Model file for the job. Use its own axes, mm. A direction names the side the tool comes from. Round coordinates to 2 decimals unless told otherwise and drop trailing zeros. Order: outer loops, then holes, each group sorted by start corner. A loop starts at its lowest first (then second) coordinate and runs counter-clockwise, first axis right, second up. Notation, with made-up numbers: (-12, 74) - (9, 74) arc R22 ccw to (9, 106) - close; hole circle Ø11 at (76, -14.75). An arc over 180 degrees is marked (long way). Put each result on its own line as item: value. Start each with the question number.
Item 1: Which spindle directions (+Z, -Z, +X, -X, +Y, -Y) get a long thin tool onto all of the face, cutting with end or side? Do faces 1 (the face through (-10, -43, -68)), 2 (the face through (-47, -27, -50)), 3 (the face through (-44.863, -37.283, 48.623)). Say none if no direction does.
Item 2: Pin check, flat tips, straight feed: pin 1 Ø5 at (x, z) = (-24, -45) entering from +Y; pin 2 Ø8 at (x, y) = (-36, -60) entering from +Z; pin 3 Ø1.5 at (x, y) = (-22.5, -65.5) entering from -Z. Stop position of each tip, or through.
Item 3: Probe probe 1 along Z at (x, y) = (-45, 2); probe 2 along X at (y, z) = (-60, -56); probe 3 along Y at (x, z) = (-3.5, -26). List the from-to ranges inside material, lowest first.
Item 4: Saw through at A-A on x = -17. List the corners of the cut face in (y, z), plus the area to 3 significant figures.
```python
from build123d import *


with BuildPart() as part:
    # OutRacSke → OuterRace (revolve)
    with BuildSketch(Plane.XY, mode=Mode.PRIVATE) as outerrace_sk:
        with BuildLine():
            Line((-10, 79.990044662), (-47, 73.1325))
            Line((-47, 73.1325), (-47, 83))
            ThreePointArc((-47, 83), (-46.414213562, 84.414213562), (-45, 85))
            Line((-45, 85), (-11.48, 85))
            Line((-11.48, 85), (-10, 83.52))
            Line((-10, 83.52), (-10, 79.990044662))
        make_face()
    revolve(outerrace_sk.sketch.rotate(Axis((-42.5, 0, 0), (1, 0, 0)), 270), axis=Axis((-42.5, 0, 0), (1, 0, 0)))

    # RolSimSke → RollersSimplified (revolve)
    with BuildSketch(Plane.XY, mode=Mode.PRIVATE) as rollerssimplified_sk:
        Polygon((-45, 73.87069398), (-12.257611578, 79.939136979), (-9.797431984, 66.665195727), (-42.539820406, 60.596752728), align=None)
    revolve(rollerssimplified_sk.sketch.rotate(Axis((0, 0, 0), (-1, 0, 0)), 90), axis=Axis((0, 0, 0), (-1, 0, 0)))

    # InsRacSke → InnerRace (revolve)
    with BuildSketch(Plane.XY, mode=Mode.PRIVATE) as innerrace_sk:
        with BuildLine():
            Line((-42.652623366, 61.271752727), (-47, 61.271752727))
            Line((-47, 61.271752727), (-47, 56.48))
            Line((-47, 56.48), (-45.52, 55))
            Line((-45.52, 55), (-2.5, 55))
            ThreePointArc((-2.5, 55), (-0.732233047, 55.732233047), (0, 57.5))
            Line((0, 57.5), (0, 68.015195726))
            Line((0, 68.015195726), (-9.785131089, 68.015195726))
            Line((-9.785131089, 68.015195726), (-9.785131089, 66.665195726))
            Line((-9.785131089, 66.665195726), (-42.527519511, 60.596752727))
            Line((-42.527519511, 60.596752727), (-42.652623366, 61.271752727))
        make_face()
    revolve(innerrace_sk.sketch.rotate(Axis((-42.5, 0, 0), (1, 0, 0)), 270), axis=Axis((-42.5, 0, 0), (1, 0, 0)))


solid = part.part
```
Results found:
1. face 1: +X
1. face 2: +Z, -Z, -X, +Y, -Y
1. face 3: -X
2. pin 1: stops at y = 73.61
2. pin 2: stops at z = 63.95
2. pin 3: stops at z = -55.07
3. probe 1: z = -84.98 to -73.48, -61.24 to -54.96, 54.96 to 61.24, 73.48 to 84.98
3. probe 2: x = -47 to -10
3. probe 3: y = -62.85 to -48.47, 48.47 to 62.85
4. outline: circle Ø170 at (0, 0); circle Ø130.66 at (0, 0); hole circle Ø130.66 at (0, 0); hole circle Ø110 at (0, 0)
4. area: 13,200 mm²
